Read the model definition and answer for the solid it produces. Units are mm, in the model's axes. A direction names the side the tool comes from. Coordinates: 2 decimals unless noted, no trailing zeros. Order: outer loops, then holes, each group sorted by start corner. A loop starts at its lowest first (then second) coordinate and runs counter-clockwise, first axis right, second up. Notation, with made-up numbers: M -28,-5.75 L 1,-5.75 A14 cw 1,4.25 Z; hole C 35.25,68 d11. An arc over 180 degrees is marked long. Use a Markdown table: item, result. Add a question column.
1) For faces 1 (the face through (-6, 11, 0)), 2 (the face through (6.5, -0.2, -1.5)), determine the directions among +Z, -Z, +X, -X, +Y, -Y from which every point of the face is accessible in a straight line to the end or side of a thin tool.
2) Find section D-D on y = -11.25. Write down the section's boundary in (x, z), plus the area to 3 significant figures.
3) The mould has two halves that part along Y. Classify faces 3 (the face through (-6, 3, 2.7)), 4 (the face through (5.96, -1.88, 0.57)), 5 (the face through (-14.985, -0.66, -0.74)): released by +Y, released by -Y, zero draft, split by the parting line, or undercut.
4) Find the intervals of material crossed by probe 1 along Y at (x, z) = (0, 0.2); probe 2 along Y at (x, z) = (0, -0.3), in increasing order. Write a range as [from, to].
5) Find section A-A on y = 0. Write down the section's boundary in (x, z), plus the area to 4 significant figures.
6) Find section C-C on z = -0.45. Write down the section's boundary in (x, y), plus the area to 3 significant figures.
7) Each of these flat-tipped pins is pushed along its axis until it touches: pin 1 Ø15 at (x, y) = (5, -3) entering from +Z; pin 2 Ø7.5 at (x, y) = (0, 0) entering from +Z; pin 3 Ø1.5 at (x, z) = (-7, 0.5) entering from +Y. Where does it stop, or does it pass through?
from build123d import *

# Parameters (mm, degrees)
F0_R     = 12.25
F1_DEPTH = 2.7
F2_R     = 15
F2_R_2   = 12.25
F3_DEPTH = 1.5
F4_R     = 6.25
F5_DEPTH = 10


with BuildPart() as f1:
    # F0 (on Top) → F1 (new body)
    with BuildSketch(Plane.XY):
        Circle(F0_R)
    extrude(amount=F1_DEPTH)

    # F2 (on face) → F3 (join)
    with BuildSketch(Plane(origin=(0, 0, 0), x_dir=(1, 0, 0), z_dir=(0, 0, -1))):
        Circle(F2_R)
        Circle(F2_R_2, mode=Mode.SUBTRACT)
        Circle(F2_R_2)
    extrude(amount=F3_DEPTH)

    # F4 (on face) → F5 (cut)
    with BuildSketch(Plane(origin=(0, 0, -1.5), x_dir=(1, 0, 0), z_dir=(0, 0, -1))):
        Circle(F4_R)
    extrude(amount=-F5_DEPTH, mode=Mode.SUBTRACT)


solid = f1.part
Check result:
| question | item | result |
|---|---|---|
| 1 | face 1 | +Z |
| 1 | face 2 | -Z, +X, -X, +Y, -Y |
| 2 | outline | M -9.92,-1.5 L 9.92,-1.5 L 9.92,0 L 4.85,0 L 4.85,2.7 L -4.85,2.7 L -4.85,0 L -9.92,0 Z |
| 2 | area | 55.9 mm2 |
| 3 | face 3 | zero draft |
| 3 | face 4 | undercut |
| 3 | face 5 | split by the parting line |
| 4 | probe 1 | y = [-12.25, -6.25], [6.25, 12.25] |
| 4 | probe 2 | y = [-15, -6.25], [6.25, 15] |
| 5 | outline | M -15,-1.5 L -6.25,-1.5 L -6.25,2.7 L -12.25,2.7 L -12.25,0 L -15,0 Z; M 6.25,-1.5 L 15,-1.5 L 15,0 L 12.25,0 L 12.25,2.7 L 6.25,2.7 Z |
| 5 | area | 58.65 mm2 |
| 6 | outline | C 0,0 d30; hole C 0,0 d12.5 |
| 6 | area | 584 mm2 |
| 7 | pin 1 | stops at z = 2.7 |
| 7 | pin 2 | passes through |
| 7 | pin 3 | stops at y = 13.55 |
